Verification items for this drawing (mm, ordinates from the low corner). A direction names the side the tool comes from. Give positions to 0.01 mm unless a question says otherwise; leave off trailing zeros. Order: outer loops, then holes, each group sorted by start corner. A loop starts at its lowest first (then second) coordinate and runs counter-clockwise, first axis right, second up. Notation, with made-up numbers: (11, 73.5) -> (33, 73.5) arc R17 ccw to (33, 100.5) -> close; hole circle Ø11 at (38.25, 16.25). An arc over 180 degrees is marked (long way). One line per question, with ' | ' between items.
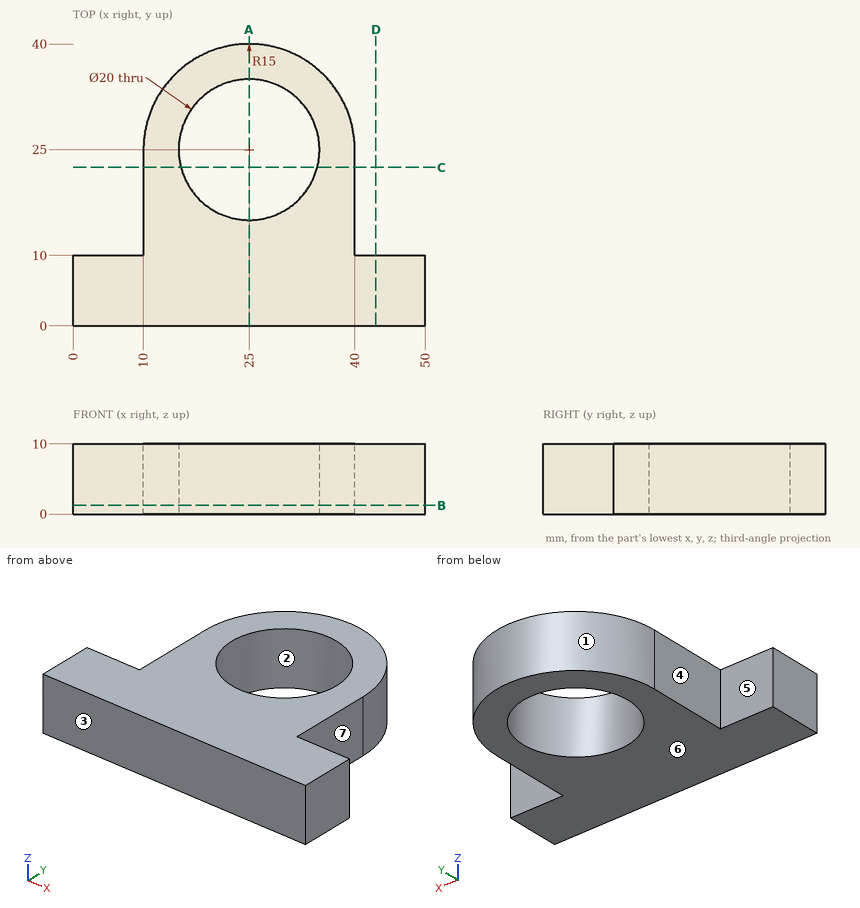
Q1. Section check B-B (z = 1.25). Enter the section's corners in (x, y).
Result sheet:
outline: (0, 0) -> (50, 0) -> (50, 10) -> (40, 10) -> (40, 25) arc R15 ccw to (10, 25) -> (10, 10) -> (0, 10) -> close; hole circle Ø20 at (25, 25)
Q2. Depth check by flat-ended pin: pin 1 Ø2 at (y, z) = (33, 5) entering from -X; pin 2 Ø1.5 at (x, z) = (27.5, 7) entering from +Y; pin 3 Ø3 at (y, z) = (17.5, 3.5) entering from -X. Enter the tip coordinate at first touch or a pass-through.
Result sheet:
pin 1: stops at x = 11.73 | pin 2: stops at y = 39.9 | pin 3: stops at x = 10
Q3. Mould release check, pull along Y, two halves, no side actions. Record for the marked faces 1, 2, 3 and 4: pulls with the +Y half, pulls with the -Y half, needs draft (parallel to the pull), parting line crosses it, or undercut.
Result sheet:
face 1: pulls with the +Y half | face 2: undercut | face 3: pulls with the -Y half | face 4: needs draft
Q4. Section check D-D (x = 43). Enter the section's corners in (y, z), and give its area (3 significant figures).
Result sheet:
outline: (0, 0) -> (10, 0) -> (10, 10) -> (0, 10) -> close | area: 100 mm2
Q5. Section check A-A (x = 25). Enter the section's corners in (y, z).
Result sheet:
outline: (0, 0) -> (15, 0) -> (15, 10) -> (0, 10) -> close; (35, 0) -> (40, 0) -> (40, 10) -> (35, 10) -> close
Q6. Access from +Z, -Z, +X, -X, +Y, -Y to the whole of each face (thin tool, end or side, straight path). Record for the marked faces 5, 6 and 7.
Result sheet:
face 5: +Z, -Z, -X, +Y | face 6: -Z, +X, -X, +Y, -Y | face 7: +Z, -Z, +X, +Y
Q7. Thickness scan on line 1 (Y direction, x = 25, z = 7); line 2 (X direction, y = 25.5, z = 7); line 3 (X direction, y = 33.5, z = 8.5). Record the ranges inside material, lowest first.
Result sheet:
line 1: y = 0 to 15, 35 to 40 | line 2: x = 10.01 to 15.01, 34.99 to 39.99 | line 3: x = 12.64 to 19.73, 30.27 to 37.36
Q8. Section check C-C (y = 22.5). Enter the section's corners in (x, z), and give its area (3 significant figures).
Result sheet:
outline: (10, 0) -> (15.32, 0) -> (15.32, 10) -> (10, 10) -> close; (34.68, 0) -> (40, 0) -> (40, 10) -> (34.68, 10) -> close | area: 106 mm2
